Check sheet for the modelled part. Datum: model origin and axes. Units: mm. A direction names the side the tool comes from. Give positions to 0.01 mm unless a question says otherwise; leave off trailing zeros. Write each loop counter-clockwise with the first axis right and the second up, starting at its lowest first coordinate (ties: lowest second). Pieces come first, ordered by that corner, then holes. Notation, with made-up numbers: (60.5, 28.25) - (103.5, 28.25) arc R12 ccw to (103.5, 45.25) - close; hole circle Ø10 at (42.25, 12.5). An arc over 180 degrees is marked (long way). Return JSON: item names as keys, results as strings. Group by question number.
```python
from build123d import *

# Parameters (mm, degrees)
BOSS_EXTRUDE1_DEPTH = 5
SKETCH2_W           = 5
SKETCH2_H           = 10
SKETCH2_W_2         = 30
SKETCH2_H_2         = 5
BOSS_EXTRUDE2_DEPTH = 45.5
SKETCH3_W           = 30
SKETCH3_H           = 15
SKETCH3_R           = 1.6
SKETCH3_W_2         = 15
SKETCH3_H_2         = 10
BOSS_EXTRUDE3_DEPTH = 5
SKETCH4_W           = 2
SKETCH4_H           = 76
SKETCH4_W_2         = 116
SKETCH4_H_2         = 2
EXTRUDE_THIN1_DEPTH = 2
SKETCH5_W           = 2
SKETCH5_H           = 47.5
EXTRUDE_THIN2_DEPTH = 2
SKETCH6_W           = 2
SKETCH6_H           = 47.5
EXTRUDE_THIN3_DEPTH = 2
SKETCH7_W           = 2
SKETCH7_H           = 47.5
EXTRUDE_THIN4_DEPTH = 2
SKETCH8_W           = 2
SKETCH8_H           = 47.5
EXTRUDE_THIN5_DEPTH = 2
RIB2_REACH          = 116.797
SKETCH9_WALL_W      = 252.8063218
SKETCH9_WALL_H      = 2
RIB3_START          = -2
RIB3_DEPTH          = 2
RIB5_REACH          = 116.797
SKETCH11_WALL_W     = 252.8063218
SKETCH11_WALL_H     = 2
RIB6_START          = -2
RIB6_DEPTH          = 2
EXTRUDE_THIN6_DEPTH = 2
SKETCH16_W          = 3.138831492
SKETCH16_H          = 8.051178831
SKETCH16_W_2        = 2.588504754
SKETCH16_H_2        = 9.327196591
CUT_EXTRUDE1_DEPTH  = 164.555036608


# Read off the part's stored shape, not the designer's step: Boss-Extrude1, Rib3, Rib6
with BuildPart() as part:
    # Boss-Extrude1 outline → Boss-Extrude1 (new body)
    with BuildSketch(Plane(origin=(0, 0, 0), x_dir=(1, 0, 0), z_dir=(0, 1, 0))):
        Polygon((19.060732093, 33), (-10.939267907, 33), (-10.939267907, 0), (-53.939267907, 0), (-53.939267907, -10), (-10.939267907, -10), (-10.939267907, -43), (19.060732093, -43), (19.060732093, -10), (62.060732093, -10), (62.060732093, 0), (19.060732093, 0), align=None)
    extrude(amount=BOSS_EXTRUDE1_DEPTH)

    # Sketch2 → Boss-Extrude2 (add)
    with BuildSketch(Plane.XZ):
        with Locations((-51.439267907, 5)):
            Rectangle(SKETCH2_W, SKETCH2_H)
        with Locations((4.060732093, 40.5)):
            Rectangle(SKETCH2_W_2, SKETCH2_H_2)
        with Locations((4.060732093, -30.5)):
            Rectangle(SKETCH2_W_2, SKETCH2_H_2)
        with Locations((59.560732093, 5)):
            Rectangle(SKETCH2_W, SKETCH2_H)
    extrude(amount=BOSS_EXTRUDE2_DEPTH)

    # Sketch3 → Boss-Extrude3 (add)
    # profile 1 of 4: a face of its own
    with BuildSketch(Plane.XZ.offset(45.5)):
        with Locations((4.060732093, 50.5)):
            Rectangle(SKETCH3_W, SKETCH3_H)
        with Locations(Location((4.060732093, 50.5, 0), (0, 0, 270))):
            Circle(SKETCH3_R, mode=Mode.SUBTRACT)
    # profile 2 of 4: a face of its own
    with BuildSketch(Plane.XZ.offset(45.5)):
        with Locations((69.560732093, 5)):
            Rectangle(SKETCH3_W_2, SKETCH3_H_2)
        with Locations(Location((69.560732093, 5, 0), (0, 0, 270))):
            Circle(SKETCH3_R, mode=Mode.SUBTRACT)
    # profile 3 of 4: a face of its own
    with BuildSketch(Plane.XZ.offset(45.5)):
        with Locations((4.060732093, -40.5)):
            Rectangle(SKETCH3_W, SKETCH3_H)
        with Locations(Location((4.060732093, -40.5, 0), (0, 0, 270))):
            Circle(SKETCH3_R, mode=Mode.SUBTRACT)
    # profile 4 of 4: a face of its own
    with BuildSketch(Plane.XZ.offset(45.5)):
        with Locations((-61.439267907, 5)):
            Rectangle(SKETCH3_W_2, SKETCH3_H_2)
        with Locations(Location((-61.439267907, 5, 0), (0, 0, 270))):
            Circle(SKETCH3_R, mode=Mode.SUBTRACT)
    extrude(amount=-BOSS_EXTRUDE3_DEPTH)

    # Sketch4 → Extrude-Thin1 (add)
    with BuildSketch(Plane(origin=(0, 5, 0), x_dir=(1, 0, 0), z_dir=(0, 1, 0))):
        with Locations((4.060732093, -5)):
            Rectangle(SKETCH4_W, SKETCH4_H)
        with Locations((4.060732093, -5)):
            Rectangle(SKETCH4_W_2, SKETCH4_H_2)
    extrude(amount=EXTRUDE_THIN1_DEPTH)

    # Sketch5 → Extrude-Thin2 (add)
    with BuildSketch(Plane.ZY.offset(53.939267907)):
        with Locations((5, -16.75)):
            Rectangle(SKETCH5_W, SKETCH5_H)
    extrude(amount=EXTRUDE_THIN2_DEPTH)

    # Sketch6 → Extrude-Thin3 (add)
    with BuildSketch(Plane(origin=(62.060732093, 0, 0), x_dir=(0, 0, -1), z_dir=(1, 0, 0))):
        with Locations((-5, -16.75)):
            Rectangle(SKETCH6_W, SKETCH6_H)
    extrude(amount=EXTRUDE_THIN3_DEPTH)

    # Sketch7 → Extrude-Thin4 (add)
    with BuildSketch(Plane.XY.offset(43)):
        with Locations((4.060732093, -16.75)):
            Rectangle(SKETCH7_W, SKETCH7_H)
    extrude(amount=EXTRUDE_THIN4_DEPTH)

    # Sketch8 → Extrude-Thin5 (add)
    with BuildSketch(Plane(origin=(0, 0, -33), x_dir=(-1, 0, 0), z_dir=(0, 0, -1))):
        with Locations((-4.060732093, -16.75)):
            Rectangle(SKETCH8_W, SKETCH8_H)
    extrude(amount=EXTRUDE_THIN5_DEPTH)

    # Sketch9 wall → Rib2 (add, up to next)
    with BuildSketch(Plane(origin=(-10.939267907, -33, 50.5), x_dir=(0, 0.707106781187, -0.707106781187), z_dir=(0, -0.707106781187, -0.707106781187)), mode=Mode.PRIVATE) as rib2_sk1:
        with Locations((0, 1)):
            Rectangle(SKETCH9_WALL_W, SKETCH9_WALL_H)
    rib2_tool1 = extrude(rib2_sk1.sketch, amount=RIB2_REACH, mode=Mode.PRIVATE) - part.part
    add(rib2_tool1.solids().sort_by_distance((-10.939267907, -33, 50.5))[0])

    # Rib3 outline → Rib3 (add)
    with BuildSketch(Plane(origin=(19.060732093, 0, 0), x_dir=(0, 0, -1), z_dir=(1, 0, 0)).offset(RIB3_START)):
        Polygon((-43, -25.5), (-58, -40.5), (-43, -40.5), align=None)
    extrude(amount=RIB3_DEPTH)

    # Sketch11 wall → Rib5 (add, up to next)
    with BuildSketch(Plane(origin=(19.060732093, -33, -40.5), x_dir=(0, 0.707106781187, 0.707106781187), z_dir=(0, -0.707106781187, 0.707106781187)), mode=Mode.PRIVATE) as rib5_sk1:
        with Locations((0, 1)):
            Rectangle(SKETCH11_WALL_W, SKETCH11_WALL_H)
    rib5_tool1 = extrude(rib5_sk1.sketch, amount=RIB5_REACH, mode=Mode.PRIVATE) - part.part
    add(rib5_tool1.solids().sort_by_distance((19.060732093, -33, -40.5))[0])

    # Rib6 outline → Rib6 (add)
    with BuildSketch(Plane.ZY.offset(10.939267907).offset(RIB6_START)):
        Polygon((-33, -25.5), (-48, -40.5), (-33, -40.5), align=None)
    extrude(amount=RIB6_DEPTH)

    # Sketch15 → Extrude-Thin6 (add)
    with BuildSketch(Plane(origin=(0, -40.5, 0), x_dir=(1, 0, 0), z_dir=(0, 1, 0))):
        Polygon((-53.468679672, -3.117647059), (-60.968679672, 0.882352941), (-61.909856142, -0.882352941), (-54.409856142, -4.882352941), align=None)
        Polygon((-54.409856142, -5.117647059), (-61.909856142, -9.117647059), (-60.968679672, -10.882352941), (-53.468679672, -6.882352941), align=None)
        Polygon((62.531320328, -4.882352941), (70.031320328, -0.882352941), (69.090143858, 0.882352941), (61.590143858, -3.117647059), align=None)
        Polygon((61.590143858, -6.882352941), (69.090143858, -10.882352941), (70.031320328, -9.117647059), (62.531320328, -5.117647059), align=None)
    extrude(amount=EXTRUDE_THIN6_DEPTH)

    # Sketch16 → Cut-Extrude1 (cut, through all)
    with BuildSketch(Plane(origin=(77.060732093, 0, 0), x_dir=(0, 0, -1), z_dir=(1, 0, 0))):
        with Locations((-11.569415746, -41.474410585)):
            Rectangle(SKETCH16_W, SKETCH16_H)
        with Locations((1.294252377, -40.836401705)):
            Rectangle(SKETCH16_W_2, SKETCH16_H_2)
    extrude(amount=-CUT_EXTRUDE1_DEPTH, mode=Mode.SUBTRACT)


solid = part.part
```
Item 1: Section check C-C on x = 29. Record the cut outline in (y, z), plus the area to 3 significant figures.
Item 2: Depth check by flat-ended pin: pin 1 (4.5 mm diameter, centred on x = 66.5, z = 3, fed in from +Y); pin 2 (1.6 mm diameter, centred on y = -6.5, z = 4.5, fed in from +X); pin 3 (16.5 mm diameter, centred on y = -34, z = 51.5, fed in from -X). Enter the tip coordinate at first touch or a pass-through.
Item 3: Access from +Z, -Z, +X, -X, +Y, -Y to the whole of each face (thin tool, end or side, straight path). Record for faces 1 (the face through (-9, 5, -10)), 2 (the face through (12, -18, -33)), 3 (the face through (57.061, -22, 5)), 4 (the face through (-51, -15, 10)), 5 (the face through (5.061, -6, 44)).
Item 4: Section check D-D on z = -9. Record the cut outline in (x, y), plus the area to 3 significant figures.
Item 5: Material ranges on line 1 along X through (y, z) = (-44, 5); line 2 along X through (y, z) = (-42.05, 50.5); line 3 along Z through (x, y) = (-8, -28.5), recorded low to high. Write a range as from..to.
Item 6: Mould release check, pull along X, two halves, no side actions. Record for faces 6 (the face through (48, 6, 4)), 7 (the face through (-58.97, -39.51, 2.45)), 8 (the face through (17.061, -36, -38)): +X half, -X half, draft (parallel to the pull), parting line (faces both ways), or undercut.
Item 7: Section check A-A on y = -20. Count the separate pieces of the cut face and the enclosed holes in it, plus the area to 3 significant figures.
Item 8: Section check B-B on z = 50.5. Record the cut outline in (x, y), plus the area to 3 significant figures.
Reply:
{
 "1": {"outline": "(0, 0) - (5, 0) - (5, 4) - (7, 4) - (7, 6) - (5, 6) - (5, 10) - (0, 10) - close", "area": "54.0 mm²"},
 "2": {"pin 1": "y = -38.5", "pin 2": "x = 64.06", "pin 3": "x = -10.94"},
 "3": {"face 1": "-Z, -X, +Y", "face 2": "-Z, +Y", "face 3": "+Z, -Z, -Y", "face 4": "+Z, -X, +Y, -Y", "face 5": "+Z, +Y"},
 "4": {"outline": "(-10.94, 0) - (19.06, 0) - (19.06, 5) - (5.06, 5) - (5.06, 7) - (3.06, 7) - (3.06, 5) - (-10.94, 5) - close", "area": "154 mm²"},
 "5": {"line 1": "-68.94..-63.04, -59.84..-48.94, 57.06..67.96, 71.16..77.06", "line 2": "-10.94..2.46, 5.66..19.06", "line 3": "-33..-28, 38..43"},
 "6": {"face 6": "draft", "face 7": "-X half", "face 8": "undercut"},
 "7": {"separate pieces": "4", "enclosed holes": "0", "area": "416 mm²"},
 "8": {"outline": "(-10.94, -45.5) - (2.46, -45.5) - (2.46, -40.5) - (-8.94, -40.5) - (-8.94, -33) - (-10.94, -33) - close; (5.66, -45.5) - (19.06, -45.5) - (19.06, -33) - (17.06, -33) - (17.06, -40.5) - (5.66, -40.5) - close", "area": "164 mm²"}
}
